from build123d import *

# Parameters (mm, degrees)
F1_DEPTH = 23
F3_DEPTH = 4.5
F5_DEPTH = 11.5
F6_R     = 6.5
F7_DEPTH = 9


with BuildPart() as f1:
    # F0 (on Top) → F1 (new body)
    with BuildSketch(Plane.XY):
        with BuildLine():
            Line((0, 114.5), (0, 0))
            Line((0, 0), (50, 0))
            Line((50, 0), (50, 100.5))
            Line((50, 100.5), (29, 100.5))
            ThreePointArc((29, 100.5), (26.171573, 101.671573), (25, 104.5))
            Line((25, 104.5), (25, 114.5))
            Line((25, 114.5), (0, 114.5))
        make_face()
    extrude(amount=F1_DEPTH)

    # F2 (on face) → F3 (cut)
    with BuildSketch(Plane.XY.offset(23)):
        with BuildLine():
            Line((41, 80), (9, 80))
            ThreePointArc((9, 80), (5, 76), (9, 72))
            Line((9, 72), (9, 14))
            ThreePointArc((9, 14), (5, 10), (9, 6))
            Line((9, 6), (41, 6))
            ThreePointArc((41, 6), (45, 10), (41, 14))
            Line((41, 14), (41, 72))
            ThreePointArc((41, 72), (45, 76), (41, 80))
        make_face()
    extrude(amount=-F3_DEPTH, mode=Mode.SUBTRACT)

    # F4 (on face) → F5 (cut)
    with BuildSketch(Plane.XY.offset(18.5)):
        with BuildLine():
            Line((9, 68), (9, 14))
            ThreePointArc((9, 14), (5, 10), (9, 6))
            Line((9, 6), (41, 6))
            ThreePointArc((41, 6), (45, 10), (41, 14))
            Line((41, 14), (41, 68))
            ThreePointArc((41, 68), (39.828427, 70.828427), (37, 72))
            Line((37, 72), (33, 72))
            Line((33, 72), (33, 76))
            ThreePointArc((33, 76), (31.828427, 78.828427), (29, 80))
            Line((29, 80), (21, 80))
            ThreePointArc((21, 80), (18.171573, 78.828427), (17, 76))
            Line((17, 76), (17, 72))
            Line((17, 72), (13, 72))
            ThreePointArc((13, 72), (10.171573, 70.828427), (9, 68))
        make_face()
    extrude(amount=-F5_DEPTH, mode=Mode.SUBTRACT)

    # F6 (on face) → F7 (cut, through all)
    with BuildSketch(Plane(origin=(0, 0, 0), x_dir=(0, -1, 0), z_dir=(-1, 0, 0))):
        with Locations((-40.5, 23)):
            Circle(F6_R)
    extrude(amount=-F7_DEPTH, mode=Mode.SUBTRACT)


solid = f1.part
Build history of the part. All positions in model axes, mm. A direction names the side the tool comes from. Give positions to 0.01 mm unless a question says otherwise; leave off trailing zeros. Order: outer loops, then holes, each group sorted by start corner. A loop starts at its lowest first (then second) coordinate and runs counter-clockwise, first axis right, second up. Notation, with made-up numbers: M 37.25,-33 L 50.25,-33 A14 ccw 50.25,-25 Z; hole C 11.25,25 d5. An arc over 180 degrees is marked long. Use one line per item in the form item = value.
1) Tool access for faces 4 (the face through (25, 109, 11)), 5 (the face through (25, 0, 11)), 6 (the face through (45, 76, 21)): list every direction of +Z, -Z, +X, -X, +Y, -Y with a clear straight run to the whole face (end or side of a thin tool).
Calculated:
face_4 = +Z, -Z, +X, +Y
face_5 = +Z, -Z, +X, -X, -Y
face_6 = +Z
2) Saw through at C-C (x = 23). Give the cut face in (y, z).
Calculated:
outline = M 0,0 L 114.5,0 L 114.5,23 L 80,23 L 80,7 L 6,7 L 6,23 L 0,23 Z
3) Saw through at D-D (z = 4). Give the cut face in (x, y), plus the area to 3 significant figures.
Calculated:
outline = M 0,0 L 50,0 L 50,100.5 L 29,100.5 A4 cw 25,104.5 L 25,114.5 L 0,114.5 Z
area = 5,380 mm2
4) Saw through at B-B (y = 58). Give the cut face in (x, z), plus the area to 3 significant figures.
Calculated:
outline = M 0,0 L 50,0 L 50,23 L 41,23 L 41,7 L 9,7 L 9,23 L 0,23 Z
area = 638 mm2
5) Saw through at A-A (z = 12.25). Give the cut face in (x, y), plus the area to 3 significant figures.
Calculated:
outline = M 0,0 L 50,0 L 50,100.5 L 29,100.5 A4 cw 25,104.5 L 25,114.5 L 0,114.5 Z; hole M 9,6 L 41,6 A4 ccw 41,14 L 41,68 A4 ccw 37,72 L 33,72 L 33,76 A4 ccw 29,80 L 21,80 A4 ccw 17,76 L 17,72 L 13,72 A4 ccw 9,68 L 9,14 A4 ccw Z
area = 3,100 mm2
6) Probe probe 1 along X at (y, z) = (49, 19); probe 2 along Y at (x, z) = (21, 22); probe 3 along Z at (x, y) = (9.5, 68.5). List the from-to ranges inside material, lowest first.
Calculated:
probe_1 = 0 to 9, 41 to 50
probe_2 = 0 to 6, 80 to 114.5
probe_3 = 0 to 7
7) Two-plate mould, pull along X, no slides. Class faces 1 (the face through (31.859, 78.797, 12.83)), 2 (the face through (50, 50, 11)), 3 (the face through (40, 100.5, 11)): released by +X, released by -X, zero draft, split by the parting line, or undercut.
Calculated:
face_1 = undercut
face_2 = released by +X
face_3 = zero draft
8) Drop flat-ended pins along their axis: pin 1 (4 mm diameter, centred on x = 35, z = 11.5, fed in from -Y); pin 2 (8 mm diameter, centred on y = 111.5, z = 15.5, fed in from +X); pin 3 (6 mm diameter, centred on x = 12.5, y = 74.5, fed in from +Z); pin 4 (2 mm diameter, centred on x = 43.5, z = 2.5, fed in from +Y). Give the stop position or say it passes through.
Calculated:
pin_1 = 0
pin_2 = 25
pin_3 = 18.5
pin_4 = 100.5
